```python
from build123d import *

# Parameters (mm, degrees)
SKETCH1_R           = 4.5
BOSS_EXTRUDE1_DEPTH = 6
SKETCH2_R           = 3
CUT_EXTRUDE1_DEPTH  = 5
SKETCH3_R           = 0.75
BOSS_EXTRUDE2_DEPTH = 4
BOSS_EXTRUDE3_DEPTH = 2
BOSS_EXTRUDE4_DEPTH = 8
SKETCH7_W           = 0.5
SKETCH7_H           = 3.5
SKETCH7_W_2         = 3.5
SKETCH7_H_2         = 0.5
BOSS_EXTRUDE5_DEPTH = 4
SKETCH8_W           = 6
SKETCH8_H           = 4
BOSS_EXTRUDE6_DEPTH = 1


with BuildPart() as part:
    # Sketch1 → Boss-Extrude1 (new body)
    with BuildSketch(Plane.XY):
        Circle(SKETCH1_R)
    extrude(amount=BOSS_EXTRUDE1_DEPTH)

    # Sketch2 → Cut-Extrude1 (cut)
    with BuildSketch(Plane.XY.offset(6)):
        Circle(SKETCH2_R)
    extrude(amount=-CUT_EXTRUDE1_DEPTH, mode=Mode.SUBTRACT)

    # Sketch3 → Boss-Extrude2 (add)
    with BuildSketch(Plane.XY.offset(1)):
        Circle(SKETCH3_R)
    extrude(amount=BOSS_EXTRUDE2_DEPTH)

    # Sketch5 → Boss-Extrude3 (add)
    with BuildSketch(Plane(origin=(0, 0, 0), x_dir=(-1, 0, 0), z_dir=(0, 0, -1))):
        with BuildLine():
            Line((-5, 6), (5, 6))
            ThreePointArc((5, 6), (5.353553391, 5.853553391), (5.5, 5.5))
            Line((5.5, 5.5), (5.5, -5.5))
            ThreePointArc((5.5, -5.5), (5.353553391, -5.853553391), (5, -6))
            Line((5, -6), (-5, -6))
            ThreePointArc((-5, -6), (-5.353553391, -5.853553391), (-5.5, -5.5))
            Line((-5.5, -5.5), (-5.5, 5.5))
            ThreePointArc((-5.5, 5.5), (-5.353553391, 5.853553391), (-5, 6))
        make_face()
    extrude(amount=BOSS_EXTRUDE3_DEPTH)

    # Sketch6 → Boss-Extrude4 (add)
    with BuildSketch(Plane(origin=(0, 0, -2), x_dir=(-1, 0, 0), z_dir=(0, 0, -1))):
        with BuildLine():
            Line((-4.5, 0), (-4.5, -6))
            Line((-4.5, -6), (4.5, -6))
            Line((4.5, -6), (4.5, 0))
            ThreePointArc((4.5, 0), (0, 4.5), (-4.5, 0))
        make_face()
    extrude(amount=BOSS_EXTRUDE4_DEPTH)

    # Sketch7 → Boss-Extrude5 (add)
    with BuildSketch(Plane(origin=(0, 0, -10), x_dir=(-1, 0, 0), z_dir=(0, 0, -1))):
        with Locations((3.672251412, -1.23876186)):
            Rectangle(SKETCH7_W, SKETCH7_H)
        with Locations((2.252036974, -5.358665001)):
            Rectangle(SKETCH7_W_2, SKETCH7_H_2)
        with Locations((-1.614241264, -2.943106028)):
            Rectangle(SKETCH7_W_2, SKETCH7_H_2)
    extrude(amount=BOSS_EXTRUDE5_DEPTH)

    # Sketch8 → Boss-Extrude6 (add)
    with BuildSketch(Plane(origin=(0, -6, 0), x_dir=(-1, 0, 0), z_dir=(0, -1, 0))):
        with Locations((-0.5, 8)):
            Rectangle(SKETCH8_W, SKETCH8_H)
    extrude(amount=BOSS_EXTRUDE6_DEPTH)


solid = part.part
```
The listing builds one solid part. Answer for the finished solid, in the listing's coordinates (mm). A direction names the side the tool comes from. Round coordinates to 2 decimals unless told otherwise and drop trailing zeros. Order: outer loops, then holes, each group sorted by start corner. A loop starts at its lowest first (then second) coordinate and runs counter-clockwise, first axis right, second up. Notation, with made-up numbers: (17.25, -21.5) - (69.25, -21.5) arc R26 ccw to (69.25, 7.5) - close; hole circle Ø1 at (-22.75, -39.75). An arc over 180 degrees is marked (long way). Put each result on its own line as item: value. Start each with the question number.
(1) For faces 4 (the flat face through (1, -1, 1)), 5 (the flat face through (-2, -5.609, -12)), 6 (the flat face through (-3.922, -1, -12)), 7 (the flat face through (-3, 4, -2)), 8 (the flat face through (0.5, -6.5, -6)), determine the directions among +Z, -Z, +X, -X, +Y, -Y from which every point of the face is accessible in a straight line to the end or side of a thin tool.
(2) Find section C-C (x = -1.75). Give the vertices of the cut face in (y, z), plus the area to 3 significant figures.
(3) Straight lines are drawn through the part: probe 1 along Y at (x, z) = (0, 3.1); probe 2 along Y at (x, z) = (0.5, 2); probe 3 along Z at (x, y) = (-4.75, -0.25). For each, find the intervals that lie inside material, in ascending order. Write a range as from..to.
(4) Find section D-D (y = 3.75). Give the vertices of the cut face in (x, z), plus the area to 3 significant figures.
(5) Find section B-B (z = -9). Give the vertices of the cut face in (x, y).
(6) Determine the mould class of faces 1 (the flat face through (3.5, -6.5, -8)), 2 (the flat face through (2, -3.193, -12)), 3 (the cylindrical face through (-3, 0, 4)) for opening direction Y: released by +Y, released by -Y, zero draft, split by the parting line, or undercut.
(7) Find section A-A (z = -11.5). Give the vertices of the cut face in (x, y), plus the area to 3 significant figures.
(8) Given P1, Ø3, axis at x = -4, z = 3.5, coming from the -Y side; P2, Ø3, axis at x = 1.5, z = -3, coming from the -Y side; P3, Ø1.8, axis at x = 1, z = -11, coming from the +Y side, each flat-ended and moving along its own axis, determine where each tip first touches the part or whether it passes through.
Reply:
1. face 4: +Z
1. face 5: -Z, +X, -X, -Y
1. face 6: -Z, -X, +Y
1. face 7: -Z, +Y
1. face 8: +Z, +X, -X, -Y
2. outline: (-7, -10) - (-5.61, -10) - (-5.61, -14) - (-5.11, -14) - (-5.11, -10) - (4.15, -10) - (4.15, -2) - (6, -2) - (6, 0) - (4.15, 0) - (4.15, 6) - (2.44, 6) - (2.44, 1) - (-2.44, 1) - (-2.44, 6) - (-4.15, 6) - (-4.15, 0) - (-6, 0) - (-6, -6) - (-7, -6) - close
2. area: 137 mm^2
3. probe 1: -4.5..-3, -0.75..0.75, 3..4.5
3. probe 2: -4.47..-2.96, -0.56..0.56, 2.96..4.47
3. probe 3: -2..0
4. outline: (-5.5, -2) - (-2.49, -2) - (-2.49, -10) - (2.49, -10) - (2.49, -2) - (5.5, -2) - (5.5, 0) - (2.49, 0) - (2.49, 6) - (-2.49, 6) - (-2.49, 0) - (-5.5, 0) - close
4. area: 91.6 mm^2
5. outline: (-4.5, -6) - (-2.5, -6) - (-2.5, -7) - (3.5, -7) - (3.5, -6) - (4.5, -6) - (4.5, 0) arc R4.5 ccw to (-4.5, 0) - close
6. face 1: zero draft
6. face 2: released by -Y
6. face 3: undercut
7. outline: (-4, -5.61) - (-0.5, -5.61) - (-0.5, -5.11) - (-4, -5.11) - close; (-3.92, -2.99) - (-3.42, -2.99) - (-3.42, 0.51) - (-3.92, 0.51) - close; (-0.14, -3.19) - (3.36, -3.19) - (3.36, -2.69) - (-0.14, -2.69) - close
7. area: 5.25 mm^2
8. P1: y = -3.74
8. P2: y = -6
8. P3: y = -2.69
